from build123d import *

# Parameters (mm, degrees)
F1_DEPTH = 38.1
F2_W     = 38.1
F2_H     = 12.7
F3_DEPTH = 38.1


with BuildPart() as f1:
    # F0 (on Front) → F1 (new body)
    with BuildSketch(Plane.XZ):
        Polygon((393.7, 0), (0, 0), (0, -12.7), (38.1, -12.7), (38.1, -25.4), (0, -25.4), (0, -38.1), (393.7, -38.1), align=None)
    extrude(amount=F1_DEPTH)

    # F2 (on face) → F3 (cut)
    with BuildSketch(Plane.XY):
        with Locations((374.65, -19.05)):
            Rectangle(F2_W, F2_H)
    extrude(amount=-F3_DEPTH, mode=Mode.SUBTRACT)


solid = f1.part
For this review, take the finished solid that the model builds, in its own axes (mm). A direction names the side the tool comes from. Coordinates: 2 decimals unless noted, no trailing zeros. Loops run counter-clockwise (first coordinate to the right, second up) from the corner with the lowest first, then second, coordinate; pieces in that order, holes last. Notation, with made-up numbers: (41, 7) - (94, 7) arc R17 cw to (94, 13) - close; hole circle Ø6 at (27.5, 31.5). An arc over 180 degrees is marked (long way). Use a Markdown table: item, result. Add a question column.
Item 1: Tool access review of faces 4 (the face through (38.1, -19, -19)), 5 (the face through (355.6, -19, -19)), 6 (the face through (0, -19, -32)): name each direction out of +Z, -Z, +X, -X, +Y, -Y from which nothing blocks a thin tool from reaching the whole face with its end or side.
Item 2: For line 1 (Z direction, x = 34, y = -26); line 2 (X direction, y = -35, z = -22); line 3 (X direction, y = -19, z = -23.5), list the stretches that pass through material, from the lowest coordinate up.
Item 3: We need section B-B (y = -30). Give the boundary of the cut face in (x, z).
Item 4: Mouldability with a two-part tool opening along Z and no side actions: class faces 1 (the face through (19, -19, -12.7)), 2 (the face through (374, -12.7, -19)), 3 (the face through (200, -19, 0)) as pulls with the +Z half, pulls with the -Z half, needs draft (parallel to the pull), parting line crosses it, or undercut.
Item 5: Insertion check: pin 1 Ø2 at (y, z) = (-14.5, -15) entering from -X. The pin has a flat end and moves straight along its axis. Give the tip position at first contact, or say it passes through.
Item 6: We need section A-A (z = -18). Give the boundary of the cut face in (x, y).
Results list:
| question | item | result |
|---|---|---|
| 1 | face 4 | -X, +Y, -Y |
| 1 | face 5 | +Z, -Z, +X |
| 1 | face 6 | +Z, -Z, -X, +Y, -Y |
| 2 | line 1 | z = -38.1 to -25.4, -12.7 to 0 |
| 2 | line 2 | x = 38.1 to 393.7 |
| 2 | line 3 | x = 38.1 to 355.6 |
| 3 | outline | (0, -38.1) - (393.7, -38.1) - (393.7, 0) - (0, 0) - (0, -12.7) - (38.1, -12.7) - (38.1, -25.4) - (0, -25.4) - close |
| 4 | face 1 | undercut |
| 4 | face 2 | needs draft |
| 4 | face 3 | pulls with the +Z half |
| 5 | pin 1 | stops at x = 38.1 |
| 6 | outline | (38.1, -38.1) - (393.7, -38.1) - (393.7, -25.4) - (355.6, -25.4) - (355.6, -12.7) - (393.7, -12.7) - (393.7, 0) - (38.1, 0) - close |
